```python
from build123d import *

# Parameters (mm, degrees)
SKETCH_R        = 10
SKETCH_R_2      = 1.5
EXTRUDE_DEPTH   = 17
SKETCH001_R     = 11.1
POCKET_DEPTH    = 7.1
SKETCH002_R     = 3.5
POCKET001_DEPTH = 11
CHAMFER_SIZE    = 1.7
POCKET002_DEPTH = 1


with BuildPart() as part:
    # Sketch → Extrude (new body)
    with BuildSketch(Plane.XY):
        with BuildLine():
            Line((-12.308851, 43.982367), (-26.621029, 1.861132))
            ThreePointArc((-26.621029, 1.861132), (-25.812964, -3.594765), (-20.907103, -6.115142))
            Line((-20.907103, -6.115142), (-16.503486, -6.115142))
            ThreePointArc((16.503486, -6.115142), (0, 17.6), (-16.503486, -6.115142))
            Line((16.503486, -6.115142), (20.907103, -6.115142))
            ThreePointArc((20.907103, -6.115142), (25.812964, -3.594765), (26.621029, 1.861132))
            Line((12.308851, 43.982367), (26.621029, 1.861132))
            ThreePointArc((12.308851, 43.982367), (0, 52.8), (-12.308851, 43.982367))
        make_face()
        with Locations((0, 39.8)):
            Circle(SKETCH_R, mode=Mode.SUBTRACT)
        with Locations((-13.85625, 21.009073)):
            Circle(SKETCH_R_2, mode=Mode.SUBTRACT)
        with Locations((13.85625, 21.009073)):
            Circle(SKETCH_R_2, mode=Mode.SUBTRACT)
        with Locations((20.7, 0)):
            Circle(SKETCH_R_2, mode=Mode.SUBTRACT)
        with Locations((-20.7, 0)):
            Circle(SKETCH_R_2, mode=Mode.SUBTRACT)
    extrude(amount=EXTRUDE_DEPTH)

    # Sketch001 → Pocket (cut)
    with BuildSketch(Plane.XY.offset(17)):
        with Locations((0, 39.8)):
            Circle(SKETCH001_R)
    extrude(amount=-POCKET_DEPTH, mode=Mode.SUBTRACT)

    # Sketch002 → Pocket001 (cut)
    with BuildSketch(Plane.XY.offset(17)):
        with Locations((-13.85625, 21.009073)):
            Circle(SKETCH002_R)
        with Locations((13.85625, 21.009073)):
            Circle(SKETCH002_R)
    extrude(amount=-POCKET001_DEPTH, mode=Mode.SUBTRACT)

    # Chamfer
    chamfer_edges = [part.edges().sort_by_distance(p)[0] for p in [
        (12.35625, 21.009073, 6),
        (-15.35625, 21.009073, 6),
    ]]
    chamfer(chamfer_edges, length=CHAMFER_SIZE)

    # Sketch003 → Pocket002 (cut)
    with BuildSketch(Plane.XY.offset(17)):
        with BuildLine():
            Line((-11.903391, 12.964154), (-23.134783, 2.651761))
            ThreePointArc((-23.134783, 2.651761), (-23.92773, -1.59429), (-20.073913, -3.54514))
            Line((-20.073913, -3.54514), (-17.331794, -3.06087))
            ThreePointArc((-11.903391, 12.964154), (-16.669564, 5.646738), (-17.331794, -3.06087))
        make_face()
        with BuildLine():
            Line((11.903391, 12.964154), (23.134782, 2.651761))
            ThreePointArc((19.479755, -3.386887), (23.779787, -1.864111), (23.134782, 2.651761))
            Line((19.479755, -3.386887), (17.339862, -3.01483))
            ThreePointArc((17.339862, -3.01483), (16.662051, 5.668868), (11.903391, 12.964154))
        make_face()
    extrude(amount=-POCKET002_DEPTH, mode=Mode.SUBTRACT)


solid = part.part
```
CAD build for the part. Positions are in the model's coordinates, mm. A direction names the side the tool comes from. Give positions to 0.01 mm unless a question says otherwise; leave off trailing zeros. Order: outer loops, then holes, each group sorted by start corner. A loop starts at its lowest first (then second) coordinate and runs counter-clockwise, first axis right, second up.
(1) Flat gauge pins, fed straight in: pin 1 (2.5 mm diameter, centred on x = 20.7, y = 0, fed in from +Z); pin 2 (2 mm diameter, centred on x = -1, z = 14.5, fed in from -Y); pin 3 (2 mm diameter, centred on y = 1.5, z = 6, fed in from -X); pin 4 (4 mm diameter, centred on x = -20.7, y = 0, fed in from +Z). Where does each tip first touch, or does it go through?
(2) Tool access for faces 1 (the flat face through (19.365, 23.217, 8.381)), 2 (the cylindrical face through (-23.956, -1.536, 16.507)): list every direction of +Z, -Z, +X, -X, +Y, -Y with a clear straight run to the whole face (end or side of a thin tool).
(3) Saw through at C-C, the plane y = 39.8. Give the cut face in (x, z), then the cut area to 3 significant figures.
(4) Saw through at D-D, the plane y = 0. Give the cut face in (x, z), then the cut area to 3 significant figures.
(5) Mould opens along Y. For faces 3 (the flat face through (0, 24, 0)), 4 (the flat face through (19, -6.115, 8)), 5 (the cylindrical face through (13.1, 17.59, 11.58)) say: released by +Y, released by -Y, zero draft, split by the parting line, or undercut.
(6) Saw through at A-A, the plane x = 2.5. Give the cut face in (y, z).
(7) Drill centre lines: L1, parallel to X at y = 0, z = 6.25; L2, parallel to Y at x = 0, z = 12.75; L3, parallel to X at y = 24, z = 16.25. Where is each one in solid material? Low to high.
(8) Saw through at B-B, the plane z = 2.25. Give the cut face in (x, y), then the cut area to 3 significant figures.
Results found:
1. pin 1: passes through
1. pin 2: stops at y = 17.49
1. pin 3: stops at x = -26.91
1. pin 4: stops at z = 16
2. face 1: +Z, -Z, +X, +Y
2. face 2: +Z
3. outline: (-13.73, 0) - (-10, 0) - (-10, 9.9) - (-11.1, 9.9) - (-11.1, 17) - (-13.73, 17) - close; (10, 0) - (13.73, 0) - (13.73, 17) - (11.1, 17) - (11.1, 9.9) - (10, 9.9) - close
3. area: 111 mm2
4. outline: (-26.94, 0) - (-22.2, 0) - (-22.2, 16) - (-24.3, 16) - (-24.3, 17) - (-26.94, 17) - close; (-19.2, 0) - (-17.6, 0) - (-17.6, 16) - (-19.2, 16) - close; (17.6, 0) - (19.2, 0) - (19.2, 16) - (17.6, 16) - close; (22.2, 0) - (26.94, 0) - (26.94, 17) - (24.3, 17) - (24.3, 16) - (22.2, 16) - close
4. area: 208 mm2
5. face 3: zero draft
5. face 4: released by -Y
5. face 5: undercut
6. outline: (17.42, 0) - (30.12, 0) - (30.12, 9.9) - (28.99, 9.9) - (28.99, 17) - (17.42, 17) - close; (49.48, 0) - (52.56, 0) - (52.56, 17) - (50.61, 17) - (50.61, 9.9) - (49.48, 9.9) - close
7. L1: x = -26.94 to -22.2, -19.2 to -17.6, 17.6 to 19.2, 22.2 to 26.94
7. L2: y = 17.6 to 28.7, 50.9 to 52.8
7. L3: x = -19.1 to -15.67, -12.04 to 12.04, 15.67 to 19.1
8. outline: (-26.62, 1.86) arc R6.03 ccw to (-20.91, -6.12) - (-16.5, -6.12) arc R17.6 cw (long way) to (16.5, -6.12) - (20.91, -6.12) arc R6.03 ccw to (26.62, 1.86) - (12.31, 43.98) arc R13 ccw to (-12.31, 43.98) - close; hole circle Ø3 at (-20.7, 0); hole circle Ø3 at (-13.86, 21.01); hole circle Ø20 at (0, 39.8); hole circle Ø3 at (13.86, 21.01); hole circle Ø3 at (20.7, 0)
8. area: 1,170 mm2
